Autodesk Inventor part; units mm, degrees
ref_plane "YZ Plane" through (0, 0, 0) normal (1, 0, 0) x (0, 1, 0)
ref_plane "XZ Plane" through (0, 0, 0) normal (0, 1, 0) x (-1, 0, 0)
ref_plane "XY Plane" through (0, 0, 0) normal (0, 0, 1) x (1, 0, 0)
sketch "Sketch1" plane through (0, 0, 0) normal (0, 0, 1) x (1, 0, 0)
  circle A0 centre (0, 0) radius 53.975 construction
  circle A1 centre (0, 0) radius 19.05
  line L0 (-100.2597, 0) -> (86.9261, 0)
  line L1 (0, -117.8456) -> (0, 102.763)
  line L2 (13.4938, 63.0969) -> (13.4937, 56.9678)
  arc A2 (-66.1831, -30.8617) -> (24.3417, -68.8486) centre (0, 0) ccw
  arc A3 (7.8581, 69.4066) -> (-23.8901, 65.6375) centre (0, 0) ccw
  arc A4 (31.2487, -44.0093) -> (17.7549, 50.9712) centre (0, 0) ccw
  arc A5 (13.4937, 56.9678) -> (17.7549, 50.9712) centre (19.8438, 56.9678) ccw
  arc A6 (13.4938, 63.0969) -> (7.8581, 69.4066) centre (7.1437, 63.0969) ccw
  line L3 (28.575, -49.1869) -> (28.575, -62.8618)
  arc A7 (24.3417, -68.8486) -> (28.575, -62.8618) centre (22.225, -62.8618) ccw
  arc A8 (31.2487, -44.0093) -> (28.575, -49.1869) centre (34.925, -49.1869) ccw
  line L4 (-61.0828, -12.5629) -> (-66.1138, -22.8801)
  arc A9 (-66.1138, -22.8801) -> (-66.1831, -30.8617) centre (-57.7807, -26.9436) ccw
  line L5 (0, 0) -> (-57.7807, -26.9436) construction
  arc A10 (-36.5638, 47.9812) -> (-59.9899, -6.35) centre (0, 0) ccw
  arc A11 (-61.0828, -12.5629) -> (-59.9899, -6.35) centre (-71.3564, -7.5532) ccw
  line L6 (-34.9493, 49.7953) -> (-27.1815, 62.9071)
  arc A12 (-36.5638, 47.9812) -> (-34.9493, 49.7953) centre (-40.4126, 53.0319) ccw
  arc A13 (-23.8901, 65.6375) -> (-27.1815, 62.9071) centre (-21.7183, 59.6705) ccw
  line L7 (0, 0) -> (-21.7183, 59.6705) construction
  point P0 (13.4937, 68.5342)
  point P1 (28.575, -45.7905)
  point P2 (28.575, -67.2021)
  point P3 (-67.9722, -26.6913)
  point P4 (-53.975, 0)
  dimension "d0" = 107.95
  dimension "d10" = 38.1
  dimension "d48" = 6.35
  dimension "d58" = 6.35
  dimension "d59" = 28.575
  dimension "d60" = 73.025
  dimension "d75" = 65
  dimension "d86" = 60.325
  dimension "d88" = 6.35
  dimension "d91" = 6.35
  dimension "d92" = 69.85
  dimension "d119" = 11.43
  dimension "d120" = 9.271
  dimension "d123" = 13.4938
  dimension "d124" = 20
  dimension "d126" = 15.24
extrude "Base" add sketch "Sketch1" along normal mid plane 6.35 contours L0 A4 A8 L3 A7 A2 L1 A1 | A1 L1 A3 A6 L2 A5 A4 L0 | A1 L0 A10 A12 L6 A13 A3 L1 | L1 A2 A9 L4 A11 A10 L0 A1
sketch "Sketch5" plane through (0, 0, 3.175) normal (0, 0, 1) x (1, 0, 0)
  circle A0 centre (0, 0) radius 19.05
  arc A1 (31.2487, -44.0093) -> (17.7549, 50.9712) centre (0, 0) ccw
  line L0 (-100.2597, 0) -> (86.9261, 0)
  line L1 (0, -117.5661) -> (0, 101.086)
  line L2 (0, 0) -> (-31.4309, 31.4309) construction
  arc A2 (-66.1831, -30.8617) -> (24.3417, -68.8486) centre (0, 0) ccw
  line L3 (31.4309, -31.4309) -> (0, 0) construction
  dimension "d49" = 45
  dimension "d50" = 44.45
  dimension "d109" = 44.45
hole "Motor Mount Hole" at (-31.4309, 31.4309, 3.175) at (31.4309, -31.4309, 3.175) direction (0, 0, -1) diameter 5.1054 end through all countersink diameter 9.779 countersink angle 82
sketch "Sketch6" plane through (0, 0, 3.175) normal (0, 0, 1) x (1, 0, 0)
  arc A0 (-66.1831, -30.8617) -> (24.3417, -68.8486) centre (0, 0) ccw
  line L0 (-99.0177, 0) -> (79.4738, 0)
  line L1 (0, -117.5661) -> (0, 101.086)
  line L2 (0, 0) -> (-21.7183, 59.6705) construction
  arc A1 (-36.5638, 47.9812) -> (-59.9899, -6.35) centre (0, 0) ccw
  line L3 (-51.0449, -37.7712) -> (0, 0) construction
  dimension "d114" = 63.5
  dimension "d121" = 63.5
  dimension "d122" = 53.5
  dimension "d127" = 20
hole "Standoffs holes to front plate" at (-51.0449, -37.7712, 3.175) at (-21.7183, 59.6705, 3.175) direction (0, 0, -1) diameter 5.1054 end through all counterbore diameter 9.779 counterbore depth 1.5875
sketch "Sketch8" plane through (0, 0, -3.175) normal (0, 0, -1) x (-1, 0, 0)
  arc A0 (23.8901, 65.6375) -> (-7.8581, 69.4066) centre (0, 0) ccw
  line L0 (91.3248, 0) -> (-78.1916, 0)
  line L1 (0, -101.8795) -> (0, 100.1019)
  line L2 (0, 0) -> (-5.5344, 63.2584) construction
  arc A1 (59.9899, -6.35) -> (36.5638, 47.9812) centre (0, 0) ccw
  line L3 (0, 0) -> (58.7006, -29.9095) construction
  point P0 (54.0079, -0.6455)
  dimension "d103" = 63.5
  dimension "d104" = 5
  dimension "d110" = 27
  dimension "d111" = 65.8812
hole "Standoff holes to back plate" at (-58.7006, -29.9095, -3.175) at (5.5344, 63.2584, -3.175) direction (0, 0, 1) diameter 5.1054 end through all counterbore diameter 9.779 counterbore depth 1.5875
sketch "Sketch7" plane through (0, 0, 3.175) normal (0, 0, 1) x (1, 0, 0)
  arc A0 (-66.1831, -30.8617) -> (24.3417, -68.8486) centre (0, 0) ccw
  arc A1 (31.2487, -44.0093) -> (17.7549, 50.9712) centre (0, 0) ccw
  arc A2 (-35.2784, -50.3828) -> (-39.1538, -55.9174) centre (-37.2161, -53.1501) ccw
  arc A3 (17.6676, -65.9365) -> (15.919, -59.4103) centre (16.7933, -62.6734) ccw
  arc A4 (-35.2784, -50.3828) -> (15.919, -59.4103) centre (0, 0) ccw
  arc A5 (-39.1538, -55.9174) -> (17.6676, -65.9365) centre (0, 0) ccw
  line L0 (-100.2597, 0) -> (86.9261, 0)
  line L1 (0, -117.5661) -> (0, 101.086)
  line L2 (16.7933, -62.6734) -> (0, 0) construction
  line L3 (0, 0) -> (-37.2161, -53.1501) construction
  dimension "d69" = 4.7625
  dimension "d70" = 6.7564
  dimension "d71" = 75
  dimension "d72" = 55
extrude "Tensioning Slot" cut sketch "Sketch7" against normal through all
sketch "Sketch10" plane through (0, 0, 3.175) normal (0, 0, 1) x (1, 0, 0)
  arc A0 (31.2487, -44.0093) -> (17.7549, 50.9712) centre (0, 0) ccw
  arc A1 (-66.1831, -30.8617) -> (24.3417, -68.8486) centre (0, 0) ccw
  line L0 (-100.2597, 0) -> (86.9261, 0)
  line L1 (0, -117.5661) -> (0, 101.086)
  arc A2 (31.6332, 37.699) -> (27.2903, 32.5233) centre (29.4617, 35.1111) ccw
  arc A3 (38.4783, -17.9427) -> (44.6017, -20.7981) centre (41.54, -19.3704) ccw
  line L2 (0, 0) -> (29.4617, 35.1111) construction
  arc A4 (44.6017, -20.7981) -> (31.6332, 37.699) centre (0, 0) ccw
  arc A5 (38.4783, -17.9427) -> (27.2903, 32.5233) centre (0, 0) ccw
  line L3 (41.54, -19.3704) -> (0, 0) construction
  dimension "d130" = 4.7625
  dimension "d131" = 6.7564
  dimension "d134" = 75
  dimension "d135" = 25
extrude "Tensioning Slot to vertical" cut sketch "Sketch10" against normal through all
properties part number "motor plate"
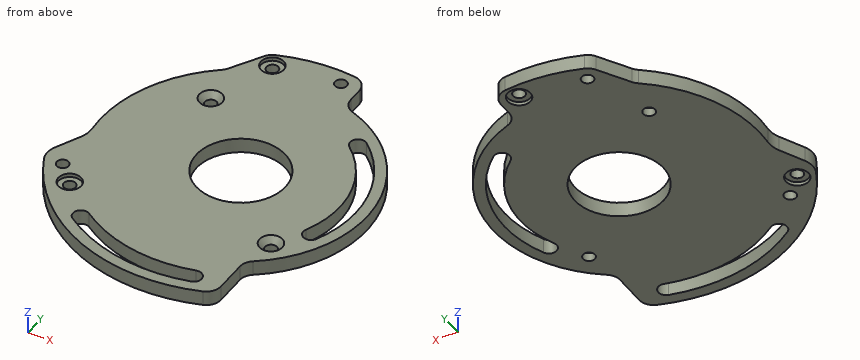
Verification items for the finished model (mm, model axes). Coordinates: 2 decimals unless noted, no trailing zeros. Order: outer loops, then holes, each group sorted by start corner. A loop starts at its lowest first (then second) coordinate and runs counter-clockwise, first axis right, second up. Notation, with made-up numbers: M 68,60 L 86,60 A24 ccw 86,96 Z; hole C 22,-38.75 d5. An arc over 180 degrees is marked long. One line per item, written item: value. Start each with the question number.
Item 1: Sectioned sample at A-A (y = 9.5). Enter the section's corners in (x, z) (3 decimals), then the cut area to 3 significant figures.
Item 2: Scan lines: probe 1 along Y at (x, z) = (-1, -3); probe 2 along Y at (x, z) = (0, 1.25); probe 3 along X at (y, z) = (32, 1). Record each from-to range of solid material in increasing order.
Item 3: Gauge pin test, flat ends, axial feed: pin 1 (8 mm diameter, centred on x = -51.04, y = -37.77, fed in from -Z) (3 decimals); pin 2 (3 mm diameter, centred on x = 5.53, y = 63.26, fed in from -Z); pin 3 (8 mm diameter, centred on x = -59, y = -30, fed in from -Z); pin 4 (3 mm diameter, centred on x = -48, z = -2, fed in from -Y). Record the tip position at first contact, or that the pin passes through.
Conclusion:
1. outline: M -59.572,-3.175 L -16.512,-3.175 L -16.512,3.175 L -59.572,3.175 Z; M 16.512,-3.175 L 41.38,-3.175 L 41.38,3.175 L 16.512,3.175 Z; M 48.287,-3.175 L 53.132,-3.175 L 53.132,3.175 L 48.287,3.175 Z
1. area: 462 mm^2
2. probe 1: y = -73.02 to -68.26, -61.5 to -19.02, 19.02 to 69.84
2. probe 2: y = -73.02 to -68.26, -61.51 to -19.05, 19.05 to 69.85
2. probe 3: x = -51.14 to -34.38, -28.49 to 27.9, 37.39 to 43.47
3. pin 1: stops at z = -3.175
3. pin 2: passes through
3. pin 3: stops at z = -1.59
3. pin 4: stops at y = -56.31
